For this review, take the finished solid that the model builds, in its own axes (mm). A direction names the side the tool comes from. Give positions to 0.01 mm unless a question says otherwise; leave off trailing zeros. Order: outer loops, then holes, each group sorted by start corner. A loop starts at its lowest first (then second) coordinate and runs counter-clockwise, first axis right, second up. Notation, with made-up numbers: (-33.75, 44.5) - (-27.75, 44.5) arc R24 cw to (-27.75, 68.5) - close; hole circle Ø7 at (-31, 9). An arc over 180 degrees is marked (long way). One line per item, written item: value.
Autodesk Inventor part; units mm, degrees
ref_plane "YZ Plane" through (0, 0, 0) normal (1, 0, 0) x (0, 1, 0)
ref_plane "XZ Plane" through (0, 0, 0) normal (0, 1, 0) x (-1, 0, 0)
ref_plane "XY Plane" through (0, 0, 0) normal (0, 0, 1) x (1, 0, 0)
ref_plane "Arbeitsebene1" through (0, 0, 0) normal (0, 0, 1) x (1, 0, 0)
sketch "Skizze1" plane through (0, 0, 0) normal (0, 0, 1) x (1, 0, 0)
  circle A0 centre (-13, -20) radius 11
  circle A1 centre (-13, -36.5) radius 2
  circle A2 centre (-13, -3.5) radius 2
  line L0 (0, 0) -> (0, -9.8388)
  line L1 (-29, 0) -> (0, 0)
  line L2 (-33, -4) -> (-29, 0)
  line L3 (-33, -4) -> (-33, -36)
  line L4 (-29, -40) -> (-33, -36)
  line L5 (0, -40) -> (-29, -40)
  line L6 (0, -30.1612) -> (0, -40)
  arc A3 (0, -30.1612) -> (0, -9.8388) centre (-13, -20) ccw
  circle A4 centre (-13, -3.5) radius 5
  circle A5 centre (-13, -36.5) radius 5
  circle A6 centre (-13, -20) radius 4.5
  line L7 (-13, -3.5) -> (-13, -36.5) construction
  line L8 (-21.5, -3.5) -> (-21.5, -36.5)
  line L9 (-4.5, -36.5) -> (-4.5, -3.5)
  arc A7 (-4.5, -3.5) -> (-21.5, -3.5) centre (-13, -3.5) ccw
  arc A8 (-21.5, -36.5) -> (-4.5, -36.5) centre (-13, -36.5) ccw
  point P0 (-13, -20)
  dimension "d0" = 10
  dimension "d1" = 10
  dimension "d2" = 9
  dimension "d3" = 17
extrude "Extrusion1" add sketch "Skizze1" along normal blind 6 contours L9 A0 L8 | A0 L8 A7 L1 A4 L9 | L9 A8 L5 A5 L8 A0 | L1 A4 A7 | A8 L5 A5
sketch "Skizze2" plane through (-21.5, -36.5, 0) normal (-1, 0, 0) x (0, 0, 1)
  line L0 (6, 21) -> (0, 21)
  line L1 (6, 12) -> (0, 12)
  circle A0 centre (3, 16.4602) radius 1.4
  point P0 (0, 36.5)
  dimension "d6" = 2.8
extrude "Extrusion2" cut sketch "Skizze2" against normal through all
sketch "Skizze3" plane through (0, 0, 6) normal (0, 0, 1) x (1, 0, 0)
  point P0 (0, 0)
sketch "Skizze4" plane through (0, 0, 6) normal (0, 0, 1) x (1, 0, 0)
  line L0 (-21.5, -3.5) -> (-21.5, -36.5)
  arc A0 (-21.5, -36.5) -> (-4.5, -36.5) centre (-13, -36.5) ccw
  line L1 (-4.5, -36.5) -> (-4.5, -3.5)
  arc A1 (-4.5, -3.5) -> (-21.5, -3.5) centre (-13, -3.5) ccw
  circle A2 centre (-13, -20) radius 4.5
  circle A3 centre (-13, -36.5) radius 5
  circle A4 centre (-13, -3.5) radius 5
  line L2 (-16, -20) -> (-11.5, -17.4019)
  line L3 (-11.5, -17.4019) -> (-11.5, -22.5981)
  line L4 (-11.5, -22.5981) -> (-16, -20)
  circle A5 centre (-13, -20) radius 1.5
  circle A6 centre (-13, -20) radius 8.5
  point P0 (0, 0)
  dimension "d9" = 3
extrude "Extrusion3" add sketch "Skizze4" against normal blind 20 contours A6 | A2
properties part number "40_XYZstage_micrometer_motorized_nema8_samplemount_lightsheet_feptube25_screwed"
(1) Wall thickness on line 1 (X direction, y = -3.5, z = 2.2); line 2 (Y direction, x = -16.25, z = 2.5); line 3 (Y direction, x = -13, z = 1.2): over which ranges is each line inside the solid? List them lowest first. Write a range as from..to.
Answers below:
line 1: x = -21.5..-18, -8..-4.5
line 2: y = -44.35..-40.3, -32.7..-7.3, 0.3..4.35
line 3: y = -45..-41.5, -31.5..-21.73, -18.27..-8.5, 1.5..5
(2) Machinability: for faces 1 (the face through (-4.5, -20, 1)), 2 (the face through (-13.718, -21.317, -3.86)), which of the approach directions +Z, -Z, +X, -X, +Y, -Y give a long, thin tool a straight path to every point of the face, cutting with its end or side? Answer none if there is none.
Answers below:
face 1: +Z, -Z, +X, +Y, -Y
face 2: +Z, -Z
(3) Take a section at D-D (z = -6.5). Write out the cut boundary in (x, y).
Answers below:
outline: circle Ø17 at (-13, -20); hole (-16, -20) - (-11.5, -22.6) - (-11.5, -17.4) - close
(4) Take a section at C-C (y = -3). Write out the cut boundary in (x, z).
Answers below:
outline: (-21.49, 0) - (-17.97, 0) - (-17.97, 6) - (-21.49, 6) - close; (-8.03, 0) - (-4.51, 0) - (-4.51, 6) - (-8.03, 6) - close
(5) Take a section at A-A (x = -17). Write out the cut boundary in (y, z), then the cut area to 3 significant figures.
Answers below:
outline: (-44, 0) - (-39.5, 0) - (-39.5, 6) - (-44, 6) - close; (-33.5, 0) - (-27.5, 0) - (-27.5, -14) - (-12.5, -14) - (-12.5, 0) - (-6.5, 0) - (-6.5, 6) - (-33.5, 6) - close; (-0.5, 0) - (4, 0) - (4, 6) - (-0.5, 6) - close
area: 426 mm^2
(6) Take a section at B-B (z = 3). Write out the cut boundary in (x, y).
Answers below:
outline: (-21.5, -36.5) arc R8.5 ccw to (-4.5, -36.5) - (-4.5, -21.44) - (-4.62, -21.44) arc R8.5 ccw to (-4.61, -18.64) - (-4.5, -18.64) - (-4.5, -3.5) arc R8.5 ccw to (-21.5, -3.5) - (-21.5, -18.64) - (-21.39, -18.64) arc R8.5 ccw to (-21.38, -21.44) - (-21.5, -21.44) - close; hole circle Ø10 at (-13, -36.5); hole circle Ø10 at (-13, -3.5); hole (-16, -20) - (-11.5, -22.6) - (-11.5, -17.4) - close
(7) Draft analysis for pull direction Y (two halves, no side actions). For faces 3 (the face through (-21.5, -20, 1)), 4 (the face through (-4.5, -20.1, 3)), 5 (the face through (-13, -45, 3)), state which applies: pulls with the +Y half, pulls with the -Y half, needs draft (parallel to the pull), parting line crosses it, or undercut.
Answers below:
face 3: needs draft
face 4: undercut
face 5: pulls with the -Y half
(8) For P1, Ø4, axis at x = -19.5, z = -0.5, coming from the -Y side; P2, Ø1.5, axis at x = -15, z = -1.5, coming from the +Y side; P3, Ø5, axis at x = -9, y = -30.5, coming from the -Z side, all flat-tipped, find the tip position at first contact; note any pin that passes through.
Answers below:
P1: stops at y = -43.67
P2: stops at y = -11.59
P3: stops at z = 0
